from build123d import *

# Parameters (mm, degrees)
BOSS_EXTRUDE1_DEPTH = 6
SKETCH2_W           = 6
SKETCH2_H           = 20
CUT_EXTRUDE1_DEPTH  = 10
SKETCH3_W           = 6
SKETCH3_H           = 20
CUT_EXTRUDE2_DEPTH  = 10
SKETCH4_W           = 20
SKETCH4_H           = 6
CUT_EXTRUDE3_DEPTH  = 10
LPATTERN1_COUNT     = 10
LPATTERN1_PITCH     = 40
SKETCH5_W           = 6
SKETCH5_H           = 20
CUT_EXTRUDE4_DEPTH  = 10


with BuildPart() as part:
    # Sketch1 → Boss-Extrude1 (new body)
    with BuildSketch(Plane.XY):
        Polygon((-114.513362239, -81.437063232), (-114.513362239, -71.437063232), (-14.513362239, -71.437063232), (265.486637761, -71.437063232), (265.486637761, -131.437063232), (-14.513362239, -131.437063232), (-114.513362239, -131.437063232), align=None)
    extrude(amount=BOSS_EXTRUDE1_DEPTH)

    # Sketch2 → Cut-Extrude1 (cut)
    with BuildSketch(Plane.XY.offset(6)):
        with Locations((-111.513362239, -101.437063232)):
            Rectangle(SKETCH2_W, SKETCH2_H)
    extrude(amount=-CUT_EXTRUDE1_DEPTH, mode=Mode.SUBTRACT)

    # Sketch3 → Cut-Extrude2 (cut)
    with BuildSketch(Plane.XY.offset(6)):
        with Locations((-17.513362239, -101.437063232)):
            Rectangle(SKETCH3_W, SKETCH3_H)
    extrude(amount=-CUT_EXTRUDE2_DEPTH, mode=Mode.SUBTRACT)

    # Sketch4 → Cut-Extrude3 (cut)
    with BuildSketch(Plane.XY.offset(6)):
        with Locations((-104.513362239, -128.437063232)):
            Rectangle(SKETCH4_W, SKETCH4_H)
    cut_extrude3 = extrude(amount=-CUT_EXTRUDE3_DEPTH, mode=Mode.SUBTRACT)

    # LPattern1: Cut-Extrude3 ×10
    with Locations(*[(i * LPATTERN1_PITCH, 0, 0) for i in range(1, LPATTERN1_COUNT)]):
        add(cut_extrude3, mode=Mode.SUBTRACT)

    # Sketch5 → Cut-Extrude4 (cut)
    with BuildSketch(Plane.XY.offset(6)):
        with Locations((262.486637761, -101.437063232)):
            Rectangle(SKETCH5_W, SKETCH5_H)
    extrude(amount=-CUT_EXTRUDE4_DEPTH, mode=Mode.SUBTRACT)


solid = part.part
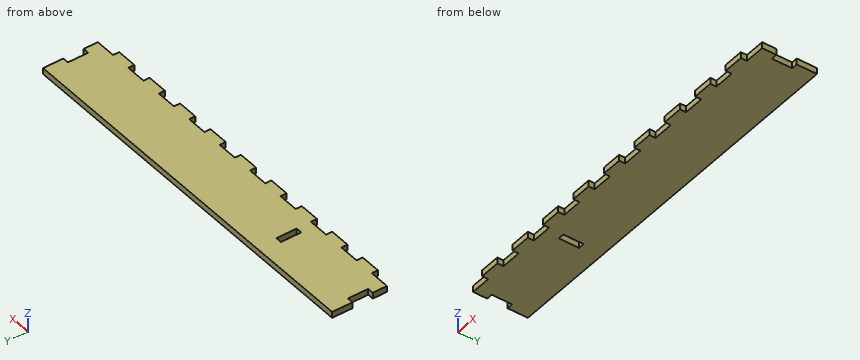
CAD build for the part. Positions are in the model's coordinates, mm. Give positions to 0.01 mm unless a question says otherwise; leave off trailing zeros. Order: outer loops, then holes, each group sorted by start corner. A loop starts at its lowest first (then second) coordinate and runs counter-clockwise, first axis right, second up. Notation, with made-up numbers: (16, 35) -> (62, 35) arc R31 cw to (62, 63) -> close; hole circle Ø11 at (-12, -11). An arc over 180 degrees is marked (long way). Return JSON: item names as keys, results as strings.
Q1. Flat gauge pins, fed straight in: pin 1 (3 mm diameter, centred on y = -128.5, z = 3.5, fed in from -X); pin 2 (1.5 mm diameter, centred on x = 178.5, z = 4, fed in from -Y); pin 3 (5 mm diameter, centred on x = 75, y = -81.5, fed in from -Z); pin 4 (3 mm diameter, centred on y = -99, z = 2.5, fed in from +X). Where does each tip first touch, or does it go through?
Working result:
{"pin 1": "x = -94.51", "pin 2": "y = -125.44", "pin 3": "z = 0", "pin 4": "x = 259.49"}
Q2. Drill centre lines: line 1 (X direction, y = -91.5, z = 1.4); line 2 (Y direction, x = -19, z = 5.5); line 3 (Y direction, x = 178, z = 2.95). Where is each one in solid material? Low to high.
Working result:
{"line 1": "-108.51 to -20.51, -14.51 to 259.49", "line 2": "-125.44 to -111.44, -91.44 to -71.44", "line 3": "-125.44 to -71.44"}
Q3. Saw through at A-A (y = -105.5). Write the cut outline in (x, z), then the cut area to 3 significant figures.
Working result:
{"outline": "(-108.51, 0) -> (-20.51, 0) -> (-20.51, 6) -> (-108.51, 6) -> close; (-14.51, 0) -> (259.49, 0) -> (259.49, 6) -> (-14.51, 6) -> close", "area": "2,170 mm²"}
Q4. Saw through at B-B (x = 220). Write the cut outline in (y, z).
Working result:
{"outline": "(-125.44, 0) -> (-71.44, 0) -> (-71.44, 6) -> (-125.44, 6) -> close"}
